For this review, take the finished solid that the model builds, in its own axes (mm). Face numbers are marked on the shaded views. Round coordinates to 2 decimals unless told otherwise and drop trailing zeros. Order: outer loops, then holes, each group sorted by start corner. A loop starts at its lowest first (then second) coordinate and runs counter-clockwise, first axis right, second up.
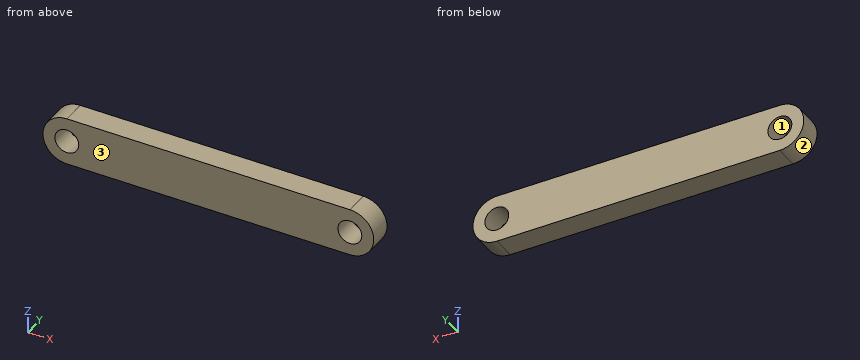
```python
from build123d import *

# Parameters (mm, degrees)
SKETCH1_R           = 1.5
BOSS_EXTRUDE1_DEPTH = 3


with BuildPart() as part:
    # Sketch1 → Boss-Extrude1 (new body)
    with BuildSketch(Plane(origin=(0, 0, 0), x_dir=(1, 0, 0), z_dir=(0, 1, 0))):
        with BuildLine():
            Line((3.344532209, 3.466749545), (-32.184472752, 3.283207502))
            ThreePointArc((-32.184472752, 3.283207502), (-35.184472752, 0.283207502), (-32.184472752, -2.716792498))
            Line((-32.184472752, -2.716792498), (-32.153477714, -2.716632379))
            Line((-32.153477714, -2.716632379), (3.375527237, -2.533090335))
            Line((3.375527237, -2.533090335), (3.406522296, -2.532930216))
            ThreePointArc((3.406522296, -2.532930216), (6.375487217, 0.482407396), (3.375527248, 3.466909665))
            Line((3.375527248, 3.466909665), (3.344532209, 3.466749545))
        make_face()
        with Locations((-32.184472752, 0.283207502)):
            Circle(SKETCH1_R, mode=Mode.SUBTRACT)
        with Locations((3.375527248, 0.466909665)):
            Circle(SKETCH1_R, mode=Mode.SUBTRACT)
    extrude(amount=BOSS_EXTRUDE1_DEPTH)


solid = part.part
```
Q1. Take a section at B-B, the plane y = 2.3. State the section outline as (x, z) points, plus the area to 3 significant figures.
Q2. Take a section at A-A, the plane z = 0.5. State the section outline as (x, y) points, plus the area to 3 significant figures.
Q3. Clearance check with a flat-ended pin moving along its axis: pin 1 (1 mm diameter, centred on x = -15.5, y = 0.5, fed in from +Z). State where the tip first meets the part, or that it passes through.
Q4. Take a section at C-C, the plane z = -1.25. State the section outline as (x, y) points.
Q5. Take a section at D-D, the plane x = -28.5. State the section outline as (y, z) points, plus the area to 3 significant figures.
Q6. Wall thickness on line 1 (X direction, y = 2.8, z = -0.5); line 2 (X direction, y = 1.85, z = 0.5); line 3 (Z direction, x = 2.5, y = 1.3): over which ranges is each line inside the solid? List them lowest first.
Q7. Mouldability with a two-part tool opening along Z and no side actions: class the marked faces 1, 2 and 3 as +Z half, -Z half, draft (parallel to the pull), parting line (faces both ways), or undercut.
Working result:
1. outline: (-32.18, -3.28) - (3.38, -3.47) arc R3 ccw to (3.41, 2.53) - (-32.18, 2.72) arc R3 ccw to start; hole circle Ø3 at (-32.18, -0.28); hole circle Ø3 at (3.38, -0.47)
1. area: 227 mm2
2. outline: (-35.08, 0) - (-33.46, 0) - (-33.46, 3) - (-35.08, 3) - close; (-30.91, 0) - (2.23, 0) - (2.23, 3) - (-30.91, 3) - close; (4.52, 0) - (6.22, 0) - (6.22, 3) - (4.52, 3) - close
2. area: 109 mm2
3. pin 1: stops at z = 2.63
4. outline: (-35.02, 0) - (-33.33, 0) - (-33.33, 3) - (-35.02, 3) - close; (-31.04, 0) - (2.1, 0) - (2.1, 3) - (-31.04, 3) - close; (4.65, 0) - (6.27, 0) - (6.27, 3) - (4.65, 3) - close
5. outline: (0, -3.3) - (3, -3.3) - (3, 2.7) - (0, 2.7) - close
5. area: 18.0 mm2
6. line 1: x = -35.18 to -33.67, -30.7 to 1.88, 4.88 to 6.38
6. line 2: x = -35.08 to -33.46, -30.91 to 2.23, 4.52 to 6.22
6. line 3: z = -3.46 to -1.68, 0.75 to 2.54
7. face 1: undercut
7. face 2: parting line
7. face 3: draft
